```python
from build123d import *

# Parameters (mm, degrees)
SKETCH_1_W         = 20
SKETCH_1_H         = 20
EXTRUDE_1_DEPTH    = 7.75
HOLE_WIZARD_M4_1_D = 3.3
HOLE_WIZARD_M4_2_D = 3.3
CHAMFER_1_SIZE     = 0.3


with BuildPart() as part:
    # 草图1 → 凸台-拉伸1 (new body, symmetric)
    with BuildSketch(Plane.XY):
        Rectangle(SKETCH_1_W, SKETCH_1_H)
    extrude(amount=EXTRUDE_1_DEPTH, both=True)

    # M4 螺纹孔1 (through all)
    with Locations(Plane.XY.offset(7.75)):
        with Locations((0, 0)):
            Hole(HOLE_WIZARD_M4_1_D / 2)

    # M4 螺纹孔2 (through all)
    with Locations(Plane(origin=(0, 10, 0), x_dir=(1, 0, 0), z_dir=(0, 1, 0))):
        with Locations((0, 0)):
            Hole(HOLE_WIZARD_M4_2_D / 2)

    # 倒角1
    chamfer_1_edges = [part.edges().sort_by_distance(p)[0] for p in [
        (-10, 0, 7.75),
        (1.65, 0, 7.75),
        (0, -10, 7.75),
        (10, 0, 7.75),
        (0, -10, -7.75),
        (-10, 0, -7.75),
        (0, 10, -7.75),
        (10, 0, -7.75),
        (10, -10, 0),
        (-10, -10, 0),
        (-10, 10, 0),
        (10, 10, 0),
        (0, 10, 7.75),
    ]]
    chamfer(chamfer_1_edges, length=CHAMFER_1_SIZE)


solid = part.part
```
Geometry: final body of the model. Coordinates: model frame, mm. Give positions to 0.01 mm unless a question says otherwise; leave off trailing zeros. Order: outer loops, then holes, each group sorted by start corner. A loop starts at its lowest first (then second) coordinate and runs counter-clockwise, first axis right, second up. Notation, with made-up numbers: M 47,53.5 L 56,53.5 A31 ccw 56,82.5 Z; hole C -34,30 d4. An arc over 180 degrees is marked long. Answer as CSV lines item,"result". Start each with the question number.
1) First-contact query: P1, Ø3, axis at x = 0, y = 0, coming from the -Z side. Flat tip, straight axial feed; report the tip coordinate or a pass-through.
2) Line query: line 1 (Z direction, x = 0, y = 7.75); line 2 (Y direction, x = 0, z = 5.25); line 3 (Y direction, x = -1, z = 3.25). Output: solid intervals per line, ascending. Write a range as from..to.
3) Cut plane A-A (y = 7.75). Output: boundary loops of the cut face in (x, z).
4) Cut plane B-B (x = 0). Output: boundary loops of the cut face in (y, z), then the cut area to 3 significant figures.
5) Mould query, pull axis X, two halves, no side actions, for faces 1 (the flat face through (-10, 0, 0)), 2 (the cylindrical face through (1.65, 0.07, 4.5)), 3 (the flat face through (-2.3, 0.1, 7.75)). Classes: +X half, -X half, draft (parallel to the pull), parting line (faces both ways), or undercut.
6) Cut plane C-C (z = 4). Output: boundary loops of the cut face in (x, y), then the cut area to 3 significant figures.
Findings below:
1,P1,"passes through"
2,line 1,"z = -7.75..-1.65, 1.65..7.75"
2,line 2,"y = -10..-1.65, 1.65..10"
2,line 3,"y = -10..-1.31, 1.31..10"
3,outline,"M -10,-7.45 L -9.7,-7.75 L 9.7,-7.75 L 10,-7.45 L 10,7.45 L 9.7,7.75 L -9.7,7.75 L -10,7.45 Z; hole C 0,0 d3.3"
4,outline,"M -10,-7.45 L -9.7,-7.75 L -1.65,-7.75 L -1.65,-1.65 L -10,-1.65 Z; M -10,1.65 L -1.65,1.65 L -1.65,7.45 L -1.95,7.75 L -9.7,7.75 L -10,7.45 Z; M 1.65,-7.75 L 9.7,-7.75 L 10,-7.45 L 10,-1.65 L 1.65,-1.65 Z; M 1.65,1.65 L 10,1.65 L 10,7.45 L 9.7,7.75 L 1.95,7.75 L 1.65,7.45 Z"
4,area,"203 mm²"
5,face 1,"-X half"
5,face 2,"undercut"
5,face 3,"draft"
6,outline,"M -10,-9.7 L -9.7,-10 L 9.7,-10 L 10,-9.7 L 10,9.7 L 9.7,10 L -9.7,10 L -10,9.7 Z; hole C 0,0 d3.3"
6,area,"391 mm²"
